from build123d import *

# Parameters (mm, degrees)
SKETCH1_W           = 180
SKETCH1_H           = 97.5
BOSS_EXTRUDE1_DEPTH = 2.5
SKETCH2_W           = 180
SKETCH2_H           = 97.5
SKETCH2_W_2         = 175
SKETCH2_H_2         = 92.5
BOSS_EXTRUDE2_DEPTH = 33
SKETCH3_W           = 180
SKETCH3_H           = 97.5
BOSS_EXTRUDE3_DEPTH = 2.5
SKETCH4_W           = 180
SKETCH4_H           = 5
BOSS_EXTRUDE4_DEPTH = 38.5
SKETCH5_W           = 180
SKETCH5_H           = 2.5
BOSS_EXTRUDE5_DEPTH = 40
SKETCH7_W           = 175
SKETCH7_H           = 33
CUT_EXTRUDE2_DEPTH  = 2.5
CUT_EXTRUDE3_DEPTH  = 2.5
SKETCH12_W          = 166
SKETCH12_H          = 31
CUT_EXTRUDE5_DEPTH  = 5
FILLET1_R           = 10
FILLET2_R           = 10
FILLET3_R           = 10
FILLET4_R           = 10


with BuildPart() as part:
    # Sketch1 → Boss-Extrude1 (new body)
    with BuildSketch(Plane.XY):
        Rectangle(SKETCH1_W, SKETCH1_H)
    extrude(amount=BOSS_EXTRUDE1_DEPTH)

    # Sketch2 → Boss-Extrude2 (add)
    with BuildSketch(Plane(origin=(0, 0, 0), x_dir=(-1, 0, 0), z_dir=(0, 0, -1))):
        Rectangle(SKETCH2_W, SKETCH2_H)
        Rectangle(SKETCH2_W_2, SKETCH2_H_2, mode=Mode.SUBTRACT)
    extrude(amount=BOSS_EXTRUDE2_DEPTH)

    # Sketch3 → Boss-Extrude3 (add)
    with BuildSketch(Plane(origin=(0, 0, -33), x_dir=(-1, 0, 0), z_dir=(0, 0, -1))):
        Rectangle(SKETCH3_W, SKETCH3_H)
    extrude(amount=BOSS_EXTRUDE3_DEPTH)

    # Sketch4 → Boss-Extrude4 (add)
    with BuildSketch(Plane(origin=(0, 0, -35.5), x_dir=(-1, 0, 0), z_dir=(0, 0, -1))):
        with Locations((0, 46.25)):
            Rectangle(SKETCH4_W, SKETCH4_H)
    extrude(amount=BOSS_EXTRUDE4_DEPTH)

    # Sketch5 → Boss-Extrude5 (add)
    with BuildSketch(Plane.XZ.offset(-43.75)):
        with Locations((0, -72.75)):
            Rectangle(SKETCH5_W, SKETCH5_H)
    extrude(amount=BOSS_EXTRUDE5_DEPTH)

    # Sketch7 → Cut-Extrude2 (cut)
    with BuildSketch(Plane(origin=(0, 48.75, 0), x_dir=(1, 0, 0), z_dir=(0, 1, 0))):
        with Locations((0, 16.5)):
            Rectangle(SKETCH7_W, SKETCH7_H)
    extrude(amount=-CUT_EXTRUDE2_DEPTH, mode=Mode.SUBTRACT)

    # Sketch9 → Cut-Extrude3 (cut)
    with BuildSketch(Plane(origin=(90, 0, 0), x_dir=(0, 0, -1), z_dir=(1, 0, 0))):
        with BuildLine():
            Line((33, 48.75), (7.5, 48.75))
            Line((7.5, 48.75), (7.5, 18.75))
            Line((7.5, 18.75), (3, 18.75))
            ThreePointArc((3, 18.75), (0.878679656, 17.871320344), (0, 15.75))
            Line((0, 15.75), (0, -15.75))
            ThreePointArc((0, -15.75), (0.878679656, -17.871320344), (3, -18.75))
            Line((3, -18.75), (7.5, -18.75))
            Line((7.5, -18.75), (7.5, -38.75))
            ThreePointArc((7.5, -38.75), (8.378679656, -40.871320344), (10.5, -41.75))
            Line((10.5, -41.75), (30, -41.75))
            ThreePointArc((30, -41.75), (32.121320344, -40.871320344), (33, -38.75))
            Line((33, -38.75), (33, 48.75))
        make_face()
    extrude(amount=-CUT_EXTRUDE3_DEPTH, mode=Mode.SUBTRACT)

    # Sketch12 → Cut-Extrude5 (cut)
    with BuildSketch(Plane(origin=(0, 48.75, 0), x_dir=(1, 0, 0), z_dir=(0, 1, 0))):
        with Locations((0, 56)):
            Rectangle(SKETCH12_W, SKETCH12_H)
    extrude(amount=-CUT_EXTRUDE5_DEPTH, mode=Mode.SUBTRACT)

    # Fillet1
    fillet1_edges = [part.edges().sort_by_distance(p)[0] for p in [
        (83, 46.25, -40.5),
    ]]
    fillet(fillet1_edges, radius=FILLET1_R)

    # Fillet2
    fillet2_edges = [part.edges().sort_by_distance(p)[0] for p in [
        (83, 46.25, -71.5),
    ]]
    fillet(fillet2_edges, radius=FILLET2_R)

    # Fillet3
    fillet3_edges = [part.edges().sort_by_distance(p)[0] for p in [
        (-83, 46.25, -40.5),
    ]]
    fillet(fillet3_edges, radius=FILLET3_R)

    # Fillet4
    fillet4_edges = [part.edges().sort_by_distance(p)[0] for p in [
        (-83, 46.25, -71.5),
    ]]
    fillet(fillet4_edges, radius=FILLET4_R)


solid = part.part
Verification items for the finished model (mm, model axes). A direction names the side the tool comes from. Coordinates: 2 decimals unless noted, no trailing zeros. Order: outer loops, then holes, each group sorted by start corner. A loop starts at its lowest first (then second) coordinate and runs counter-clockwise, first axis right, second up. Notation, with made-up numbers: (67.25, 13.25) -> (82.25, 13.25) arc R3 ccw to (82.25, 17.25) -> close; hole circle Ø11 at (-3.5, -32.75). An arc over 180 degrees is marked (long way). Put each result on its own line as item: value. Start each with the question number.
1. Material ranges on L1, parallel to Z at x = -65, y = 10; L2, parallel to Z at x = -28, y = -19.5; L3, parallel to Y at x = 55.5, z = -16, recorded low to high. Write a range as [from, to].
2. Go/stop test with flat-tipped pins: pin 1 Ø10 at (y, z) = (-9.5, -16) entering from +X; pin 2 Ø2 at (x, z) = (-60, -41) entering from -Y; pin 3 Ø3 at (x, z) = (12, -72.5) entering from -Y. Record where each tip stops, or that it passes through.
3. Cross-section at A-A, the plane y = 37. Record the boundary of the cut face in (x, z), then the cut area to 3 significant figures.
4. Cross-section at B-B, the plane z = -64. Record the boundary of the cut face in (x, y), then the cut area to 3 significant figures.
5. Cross-section at C-C, the plane x = 27. Record the boundary of the cut face in (y, z).
6. Mould release check, pull along Z, two halves, no side actions. Record for faces 1 (the flat face through (-1, 1, 2.5)), 2 (the flat face through (0, 43.75, -40)), 3 (the flat face through (1, -48.75, -16)): released by +Z, released by -Z, zero draft, split by the parting line, or undercut.
7. Access from +Z, -Z, +X, -X, +Y, -Y to the whole of each face (thin tool, end or side, straight path). Record for faces 4 (the flat face through (1, -2, -35.5)), 5 (the flat face through (1, -46.25, -16)), 6 (the flat face through (-1, 46, -40.5)).
8. Cross-section at D-D, the plane y = -28. Record the boundary of the cut face in (x, z).
Computed:
1. L1: [-74, -71.5], [-35.5, -33], [0, 2.5]
1. L2: [-35.5, -33], [0, 2.5]
1. L3: [-48.75, -46.25]
2. pin 1: x = -87.5
2. pin 2: y = 43.75
2. pin 3: y = 3.75
3. outline: (-90, -74) -> (90, -74) -> (90, -71.5) -> (-90, -71.5) -> close; (-90, -35.5) -> (90, -35.5) -> (90, -33) -> (-87.5, -33) -> (-87.5, 0) -> (87.5, 0) -> (87.5, -7.5) -> (90, -7.5) -> (90, 2.5) -> (-90, 2.5) -> close
3. area: 1,450 mm2
4. outline: (-90, 43.75) -> (-82.68, 43.75) -> (-82.68, 48.75) -> (-90, 48.75) -> close; (82.68, 43.75) -> (90, 43.75) -> (90, 48.75) -> (82.68, 48.75) -> close
4. area: 73.2 mm2
5. outline: (-48.75, -35.5) -> (43.75, -35.5) -> (43.75, -40.5) -> (48.75, -40.5) -> (48.75, -33) -> (-46.25, -33) -> (-46.25, 0) -> (48.75, 0) -> (48.75, 2.5) -> (-48.75, 2.5) -> close; (3.75, -74) -> (48.75, -74) -> (48.75, -71.5) -> (3.75, -71.5) -> close
6. face 1: released by +Z
6. face 2: undercut
6. face 3: zero draft
7. face 4: +X, -X, -Y
7. face 5: +Y
7. face 6: +Y, -Y
8. outline: (-90, -35.5) -> (90, -35.5) -> (90, -33) -> (-87.5, -33) -> (-87.5, 0) -> (87.5, 0) -> (87.5, -7.5) -> (90, -7.5) -> (90, 2.5) -> (-90, 2.5) -> close
